Geometry check sheet. Reference: drawing and pictorial views, mm from the part's lowest x, y, z. A direction names the side the tool comes from. Coordinates: 2 decimals unless noted, no trailing zeros. Order: outer loops, then holes, each group sorted by start corner. A loop starts at its lowest first (then second) coordinate and runs counter-clockwise, first axis right, second up. Notation, with made-up numbers: M 39,10.5 L 84,10.5 A23 cw 84,36.5 Z; hole C -37,33.5 d6. An arc over 180 degrees is marked long. Return JSON: item names as keys, results as strings.
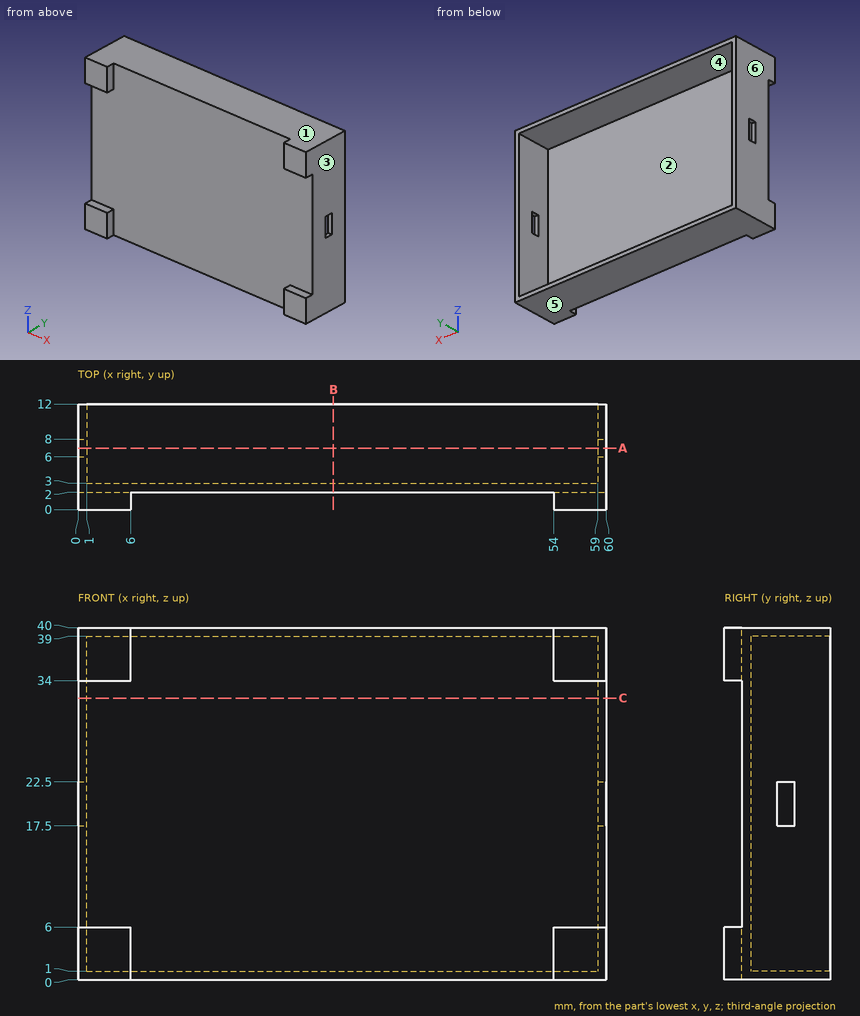
Q1. Draft check along X on the marked faces 3, 4, 5 and 6. Enter one of: pulls with the +X half, pulls with the -X half, needs draft (parallel to the pull), parting line crosses it, or undercut.
Values:
{"face 3": "pulls with the +X half", "face 4": "undercut", "face 5": "needs draft", "face 6": "pulls with the -X half"}
Q2. Cross-section at B-B, the plane x = 29. Record the boundary of the cut face in (y, z).
Values:
{"outline": "M 2,0 L 12,0 L 12,1 L 3,1 L 3,39 L 12,39 L 12,40 L 2,40 Z"}
Q3. Tool access check on the marked faces 1 and 2. Record the directions out of +Z, -Z, +X, -X, +Y, -Y that give a thin tool (end or side, any length) a straight path to the whole face; none if there is none.
Values:
{"face 1": "+Z, +X, -X, +Y, -Y", "face 2": "+Y"}
Q4. Cross-section at C-C, the plane z = 32. Record the boundary of the cut face in (x, y), and give its area (3 significant figures).
Values:
{"outline": "M 0,2 L 60,2 L 60,12 L 59,12 L 59,3 L 1,3 L 1,12 L 0,12 Z", "area": "78.0 mm^2"}
Q5. Go/stop test with flat-tipped pins: pin 1 (1.5 mm diameter, centred on x = 12.5, z = 16, fed in from +Y); pin 2 (20 mm diameter, centred on x = 28.5, z = 28.5, fed in from -Y). Record where each tip stops, or that it passes through.
Values:
{"pin 1": "y = 3", "pin 2": "y = 2"}
Q6. Cross-section at A-A, the plane y = 7. Record the boundary of the cut face in (x, z), and give its area (3 significant figures).
Values:
{"outline": "M 0,0 L 60,0 L 60,17.5 L 59,17.5 L 59,1 L 1,1 L 1,17.5 L 0,17.5 Z; M 0,22.5 L 1,22.5 L 1,39 L 59,39 L 59,22.5 L 60,22.5 L 60,40 L 0,40 Z", "area": "186 mm^2"}
Q7. Material ranges on line 1 along Z through (x, y) = (41, 9); line 2 along X through (y, z) = (4.5, 21); line 3 along Z through (x, y) = (54.5, 1.5), recorded low to high.
Values:
{"line 1": "0 to 1, 39 to 40", "line 2": "0 to 1, 59 to 60", "line 3": "0 to 6, 34 to 40"}
